Read the model definition and answer for the solid it produces. Units are mm, in the model's axes. A direction names the side the tool comes from. Coordinates: 2 decimals unless noted, no trailing zeros. Order: outer loops, then holes, each group sorted by start corner. A loop starts at its lowest first (then second) coordinate and runs counter-clockwise, first axis right, second up. Notation, with made-up numbers: M -1,43 L 33,43 A29 cw 33,69 Z; hole C 70.25,40.5 d11. An arc over 180 degrees is marked long. Use a Markdown table: item, result. Add a question column.
1) Find the intervals of material crossed by probe 1 along X at (y, z) = (3.25, 0); probe 2 along X at (y, z) = (3.75, 3.25); probe 3 along Z at (x, y) = (3.25, 4), in increasing order. Write a range as [from, to].
2) Find section B-B on x = 2.5. Write down the section's boundary in (y, z), plus the area to 3 significant figures.
3) Each of these flat-tipped pins is pushed along its axis until it touches: pin 1 Ø3.5 at (x, z) = (4.5, 2) entering from +Y; pin 2 Ø1.5 at (x, z) = (-1.5, 6.5) entering from +Y; pin 3 Ø1 at (x, y) = (5, 10) entering from +Z; pin 4 Ø5 at (x, z) = (-1, -0.5) entering from +Y. Where does it stop, or does it pass through?
4) Find section A-A on y = 4. Write down the section's boundary in (x, z), plus the area to 3 significant figures.
5) Find section C-C on z = -2.25. Write down the section's boundary in (x, y).
6) Find section D-D on y = 9. Write down the section's boundary in (x, z).
7) The mould has two halves that part along Z. Classify faces 4 (the face through (0, 6.5, 0)), 5 (the face through (6, 6.5, 3)), 6 (the face through (-3.2, 3.2, -5.66)): released by +Z, released by -Z, zero draft, split by the parting line, or undercut.
8) For faces 1 (the face through (-6, 6.5, 3)), 2 (the face through (-3.905, 3.204, 0.867)), 3 (the face through (6, 6.5, -3)), determine the directions among +Z, -Z, +X, -X, +Y, -Y from which every point of the face is accessible in a straight line to the end or side of a thin tool.
from build123d import *

# Parameters (mm, degrees)
EXTRUDE_1_DEPTH     = 6.5
SKETCH_6_R          = 4
CUT_EXTRUDE_1_DEPTH = 6.5


with BuildPart() as part:
    # ｽｹｯﾁ1 → ﾎﾞｽ - 押し出し1 (new body)
    with BuildSketch(Plane(origin=(0, 0, 0), x_dir=(1, 0, 0), z_dir=(0, 1, 0))):
        Polygon((0, -7.505553499), (6.5, -3.75277675), (6.5, 3.75277675), (0, 7.505553499), (-6.5, 3.75277675), (-6.5, -3.75277675), align=None)
    extrude(amount=EXTRUDE_1_DEPTH)

    # ｽｹｯﾁ5 → 回転1 (revolve)
    with BuildSketch(Plane.XY):
        with BuildLine():
            Line((0, 13), (0, 6.5))
            Line((0, 6.5), (6.5, 6.5))
            ThreePointArc((6.5, 6.5), (4.596194078, 11.096194078), (0, 13))
        make_face()
    revolve(axis=Axis((0, 13, 0), (0, -1, 0)))

    # ｽｹｯﾁ6 → ｶｯﾄ - 押し出し1 (cut)
    with BuildSketch(Plane.XZ):
        with Locations(Location((0, 0, 0), (0, 0, 270))):
            Circle(SKETCH_6_R)
    extrude(amount=-CUT_EXTRUDE_1_DEPTH, mode=Mode.SUBTRACT)


solid = part.part
Check result:
| question | item | result |
|---|---|---|
| 1 | probe 1 | x = [-6.5, -4], [4, 6.5] |
| 1 | probe 2 | x = [-6.5, -2.33], [2.33, 6.5] |
| 1 | probe 3 | z = [-5.63, -2.33], [2.33, 5.63] |
| 2 | outline | M 0,-6.06 L 6.5,-6.06 L 6.5,-6 A6 ccw 6.5,6 L 6.5,6.06 L 0,6.06 L 0,3.12 L 6.5,3.12 L 6.5,-3.12 L 0,-3.12 Z |
| 2 | area | 94.8 mm2 |
| 3 | pin 1 | stops at y = 12.17 |
| 3 | pin 2 | stops at y = 9.18 |
| 3 | pin 3 | stops at z = 3.29 |
| 3 | pin 4 | stops at y = 13 |
| 4 | outline | M -6.5,-3.75 L 0,-7.51 L 6.5,-3.75 L 6.5,3.75 L 0,7.51 L -6.5,3.75 Z; hole C 0,0 d8 |
| 4 | area | 96.1 mm2 |
| 5 | outline | M -6.5,0 L -3.31,0 L -3.31,6.5 L 3.31,6.5 L 3.31,0 L 6.5,0 L 6.5,6.5 L 6.1,6.5 A6.1 ccw -6.1,6.5 L -6.5,6.5 Z |
| 6 | outline | C 0,0 d12 |
| 7 | face 4 | undercut |
| 7 | face 5 | zero draft |
| 7 | face 6 | released by -Z |
| 8 | face 1 | +Z, -X, +Y |
| 8 | face 2 | -Y |
| 8 | face 3 | -Z, +X, +Y |
